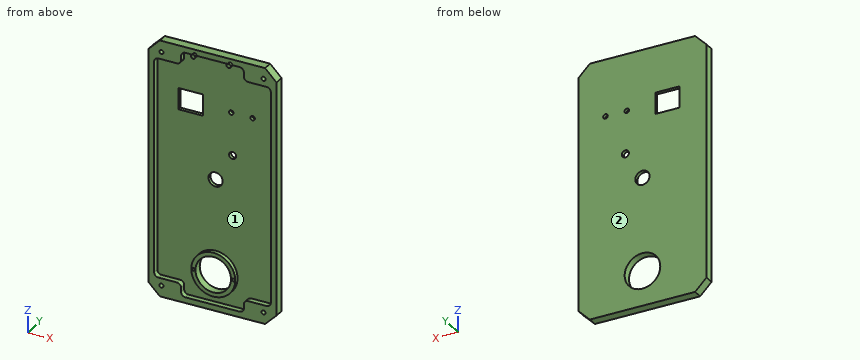
Autodesk Inventor part; units mm, degrees
ref_plane "Work Plane2" through (0, -4, 0) normal (0, -1, 0) x (1, 0, 0)
ref_plane "Work Plane1" through (0, -4, 0) normal (0, -1, 0) x (1, 0, 0)
ref_plane "YZ Plane" through (0, 0, 0) normal (1, 0, 0) x (0, 1, 0)
sketch "Sketch1" plane through (0, 0, 0) normal (0, 1, 0) x (-1, 0, 0)
  line L0 (37, -90) -> (-37, -90)
  line L1 (-45, -82) -> (-45, 82)
  line L2 (-37, 90) -> (37, 90)
  line L3 (45, 82) -> (45, -82)
  line L4 (45, -90) -> (-45, 90) construction
  line L5 (-45, -90) -> (45, 90) construction
  line L6 (-37, -90) -> (-45, -82)
  line L7 (37, -90) -> (45, -82)
  line L8 (37, 90) -> (45, 82)
  line L9 (-45, 82) -> (-37, 90)
  line L10 (0, 0) -> (0, -65.5)
  circle A0 centre (0, -65.5) radius 12.5
  line L11 (0, 0) -> (0, 0)
  circle A1 centre (0, 0) radius 5
  line L12 (0, 0) -> (17.5, 0)
  line L13 (17.5, 0) -> (17.5, 50)
  line L14 (17.5, 50) -> (0, 50)
  line L15 (0, 50) -> (0, 0)
  line L16 (26, 42.5) -> (9, 42.5)
  line L17 (9, 42.5) -> (9, 57.5)
  line L18 (9, 57.5) -> (26, 57.5)
  line L19 (26, 57.5) -> (26, 42.5)
  line L20 (26, 42.5) -> (9, 57.5) construction
  line L21 (9, 42.5) -> (26, 57.5) construction
  line L22 (9, 50) -> (-11, 50)
  circle A2 centre (-11, 50) radius 1.6
  line L23 (-11, 50) -> (-26, 50)
  circle A3 centre (-26, 50) radius 1.6
  line L24 (41, -80.3431) -> (35.3431, -86)
  line L25 (35.3431, -86) -> (-35.3431, -86)
  line L26 (-35.3431, -86) -> (-41, -80.3431)
  line L27 (-41, -80.3431) -> (-41, 80.3431)
  line L28 (-41, 80.3431) -> (-35.3431, 86)
  line L29 (-35.3431, 86) -> (35.3431, 86)
  line L30 (35.3431, 86) -> (41, 80.3431)
  line L31 (41, 80.3431) -> (41, -80.3431)
  line L32 (45, -90) -> (35.8917, -82.1873)
  circle A4 centre (35.8917, -82.1873) radius 1.45
  circle A5 centre (35.8917, -82.1873) radius 4.45
  line L33 (22.0647, -90) -> (45, -90)
  line L34 (45, -90) -> (45, -77.0647)
  line L35 (45, -77.0647) -> (22.0647, -77.0647)
  line L36 (22.0647, -77.0647) -> (22.0647, -90)
  circle A6 centre (-35.8917, -82.1873) radius 1.45
  circle A7 centre (-35.8917, -82.1873) radius 4.45
  line L37 (-45, -77.0647) -> (-22.0647, -77.0647)
  line L38 (-22.0647, -77.0647) -> (-22.0647, -90)
  circle A8 centre (35.8917, 82.1873) radius 1.45
  circle A9 centre (35.8917, 82.1873) radius 4.45
  line L39 (45, 77.0647) -> (22.0647, 77.0647)
  line L40 (22.0647, 77.0647) -> (22.0647, 90)
  circle A10 centre (-35.8917, 82.1873) radius 4.45
  circle A11 centre (-35.8917, 82.1873) radius 1.45
  line L41 (-45, 77.0647) -> (-22.0647, 77.0647)
  line L42 (-22.0647, 77.0647) -> (-22.0647, 90)
  line L43 (-22.0647, -90) -> (-45, -90)
  line L44 (-45, -90) -> (-45, -77.0647)
  line L45 (-22.0647, 90) -> (-45, 90)
  line L46 (-45, 90) -> (-45, 77.0647)
  line L47 (22.0647, 90) -> (45, 90)
  line L48 (45, 90) -> (45, 77.0647)
  line L49 (0, 0) -> (0, 20)
  line L50 (0, 0) -> (20, 0) construction
  line L51 (0, 20) -> (-12, 20)
  circle A12 centre (-12, 20) radius 2.5
  line L52 (0, 86) -> (12.5, 86)
  line L53 (0, 86) -> (-12.5, 86)
  circle A13 centre (12.5, 86) radius 1.5
  circle A14 centre (-12.5, 86) radius 1.5
  line L54 (0, -65.5) -> (14, -65.5)
  line L55 (0, -65.5) -> (14, -65.5) construction
  line L56 (0, -65.5) -> (-14, -65.5)
  line L57 (0, -65.5) -> (14, -65.5) construction
  circle A15 centre (14, -65.5) radius 0.95
  circle A16 centre (-14, -65.5) radius 0.95
  circle A17 centre (0, -65.5) radius 15.45
  point P0 (22.0647, -86)
  point P1 (-22.0647, -86)
  point P2 (-22.0647, -81.5147)
  point P3 (-26.5147, -77.0647)
  point P4 (-41, -77.0647)
  point P5 (-41, 77.0647)
  point P6 (-26.5147, 77.0647)
  point P7 (-22.0647, 81.5147)
  point P8 (-22.0647, 86)
  point P9 (22.0647, 86)
  point P10 (22.0647, 81.5147)
  point P11 (26.5147, 77.0647)
  point P12 (41, 77.0647)
  point P13 (41, -77.0647)
  point P14 (26.5147, -77.0647)
  point P15 (22.0647, -81.5147)
  point P16 (5, 0)
  point P17 (0, 5)
  point P18 (9, 50)
  point P19 (17.5, 42.5)
  dimension "d0" = 90
  dimension "d1" = 180
  dimension "d2" = 8
  dimension "d3" = 8
  dimension "d4" = 8
  dimension "d5" = 8
  dimension "d6" = 8
  dimension "d7" = 8
  dimension "d8" = 8
  dimension "d9" = 8
  dimension "d10" = 65.5
  dimension "d11" = 25
  dimension "d12" = 0
  dimension "d13" = 10
  dimension "d14" = 17.5
  dimension "d15" = 50
  dimension "d16" = 17
  dimension "d17" = 15
  dimension "d20" = 20
  dimension "d21" = 3.2
  dimension "d22" = 15
  dimension "d23" = 3.2
  dimension "d24" = 4
  dimension "d25" = 12
  dimension "d26" = 2.9
  dimension "d27" = 3
  dimension "d57" = 20
  dimension "d58" = 90
  dimension "d59" = 12
  dimension "d60" = 90
  dimension "d61" = 5
  dimension "d70" = 12.5
  dimension "d71" = 12.5
  dimension "d72" = 3
  dimension "d73" = 3
  dimension "d74" = 14
  dimension "d75" = 0
  dimension "d76" = 14
  dimension "d77" = 180
  dimension "d78" = 1.9
  dimension "d79" = 1.9
  dimension "d80" = 30.9
extrude "Extrusion1" add sketch "Sketch1" along normal blind 2.5 contours L0 L36 L25 A5 L32 L7 | L0 L38 L25 L36 | L32 A5 L24 L31 L35 L3 L7 | L0 L6 L1 L37 L27 L26 A7 L25 L38 | L36 L35 L31 L24 A5 L25 | L25 L38 L37 L27 L41 L42 L29 A14 A13 L40 L39 L31 L35 L36 | A5 L25 L24 L32 | L32 L24 A5 | L25 A7 L26 L27 L37 L38 | A4 | A5 L24 L25 | L35 L31 L39 L3 | A7 L26 L25 | L25 L26 A7 | L39 L31 L30 A9 L29 L40 L2 L8 L3 | L1 L41 L27 L37 | L39 L40 L29 A9 L30 L31 | L1 L9 L2 L42 L29 A10 L28 L27 L41 | L27 L28 A10 L29 L42 L41 | A9 L29 L30 | L30 L29 A9 | L29 A13 A14 L42 L2 L40 | A10 L29 L28 | L28 L29 A10 | A13 L29 | L29 A13 | A14 L29 | L29 A14 | A15 | A16 | A17 | A12 | A1 L15 L14 L17 L16 L13 L12 | A6 | A8 | A11
sketch "Sketch2" plane through (0, 0, 0) normal (0, -1, 0) x (1, 0, 0)
  line L0 (-26, 57.5) -> (-26, 42.5)
  line L1 (-26, 50) -> (-5, 50)
  circle A0 centre (-5, 50) radius 1.45
  circle A1 centre (-5, 50) radius 3.45
  circle A2 centre (0, -65.5) radius 12.5
  line L2 (0, -65.5) -> (-14, -65.5)
  line L3 (0, -65.5) -> (14, -65.5)
  circle A3 centre (-14, -65.5) radius 0.95
  circle A4 centre (14, -65.5) radius 0.95
  circle A5 centre (-14, -65.5) radius 1.45
  circle A6 centre (14, -65.5) radius 1.45
  line L4 (-14, -66.95) -> (-12.3751, -67.2629) construction
  line L5 (-12.3751, -67.2629) -> (-11.6091, -68.4979) construction
  spline S0 degree 2 poles (-14, -66.95) (-12.3751, -67.2629) (-11.6091, -68.4979) knots 1 1 1 2 2 2
  line L6 (-14, -64.05) -> (-12.3751, -63.7371) construction
  line L7 (-12.3751, -63.7371) -> (-11.6091, -62.5021) construction
  spline S1 degree 2 poles (-14, -64.05) (-12.3751, -63.7371) (-11.6091, -62.5021) knots 1 1 1 2 2 2
  line L8 (0, -65.5) -> (0, -61.9317)
  line L9 (14, -66.95) -> (12.3751, -67.2629) construction
  line L10 (12.3751, -67.2629) -> (11.6091, -68.4979) construction
  spline S2 degree 2 poles (14, -66.95) (12.3751, -67.2629) (11.6091, -68.4979) knots 1 1 1 2 2 2
  spline S3 degree 2 poles (14, -64.05) (12.3751, -63.7371) (11.6091, -62.5021) knots 1 1 1 2 2 2
  line L11 (14, -64.05) -> (12.3751, -63.7371) construction
  line L12 (12.3751, -63.7371) -> (11.6091, -62.5021) construction
  circle A7 centre (0, -65.5) radius 12.5
  line L13 (-22.0647, 86) -> (22.0647, 86)
  line L14 (0, 60) -> (12.5, 60)
  line L15 (12.5, 60) -> (12.5, 86)
  line L16 (12.5, 86) -> (0, 86)
  line L17 (0, 86) -> (0, 60)
  circle A8 centre (12.5, 86) radius 1.5
  circle A9 centre (-12.5, 86) radius 1.5
  circle A10 centre (0, -65.5) radius 15.45
  point P0 (0, 0)
  point P1 (-12.3047, -67.7011)
  point P2 (-12.3047, -63.2989)
  point P3 (14, -64.05)
  point P4 (12.3047, -63.2989)
  point P5 (12.3047, -67.7011)
  point P6 (-15.45, -65.5)
  point P7 (15.45, -65.5)
  dimension "d30" = 21
  dimension "d31" = 2.9
  dimension "d32" = 2
  dimension "d33" = 14
  dimension "d34" = 14
  dimension "d35" = 1.9
  dimension "d36" = 1.9
  dimension "d37" = 0.5
  dimension "d38" = 0.5
  dimension "d41" = 12.5
  dimension "d42" = 3
ref_plane "Work Plane2" through (0, -4, 0) normal (0, -1, 0) x (1, 0, 0)
sketch "Sketch4" plane through (0, -4, 0) normal (0, -1, 0) x (1, 0, 0)
  line L0 (40.0685, -6.5) -> (29.9315, -6.5)
  line L1 (29.9315, -6.5) -> (29.9315, 6.5)
  line L2 (29.9315, 6.5) -> (40.0685, 6.5)
  line L3 (40.0685, 6.5) -> (40.0685, -6.5)
  line L4 (35, 82) -> (35, -82)
  line L5 (40.0685, -6.5) -> (29.9315, 6.5) construction
  line L6 (29.9315, -6.5) -> (40.0685, 6.5) construction
  point P0 (0, 0)
  point P1 (35, 0)
  point P2 (35, -6.5)
  point P3 (35, 6.5)
  dimension "d49" = 13
ref_plane "Work Plane1" through (0, -4, 0) normal (0, -1, 0) x (1, 0, 0)
sketch "Sketch5" plane through (0, -4, 0) normal (0, -1, 0) x (1, 0, 0)
  circle A0 centre (26.5147, -81.5147) radius 1.45
  circle A1 centre (26.5147, -81.5147) radius 1.45
  circle A2 centre (-26.5147, -81.5147) radius 1.45
  circle A3 centre (-26.5147, -81.5147) radius 1.45
  circle A4 centre (26.5147, 81.5147) radius 1.45
  circle A5 centre (26.5147, 81.5147) radius 1.45
  circle A6 centre (-26.5147, 81.5147) radius 1.45
  circle A7 centre (-26.5147, 81.5147) radius 1.45
  point P0 (0, 0)
extrude "Extrusion8" add sketch "Sketch1" against normal blind 4 contours L0 L36 L25 A5 L32 L7 | L0 L38 L25 L36 | L32 A5 L24 L31 L35 L3 L7 | L0 L6 L1 L37 L27 L26 A7 L25 L38 | L36 L35 L31 L24 A5 L25 | A5 L25 L24 L32 | L32 L24 A5 | L25 A7 L26 L27 L37 L38 | A5 L24 L25 | L35 L31 L39 L3 | A7 L26 L25 | L25 L26 A7 | L39 L31 L30 A9 L29 L40 L2 L8 L3 | L1 L41 L27 L37 | L39 L40 L29 A9 L30 L31 | L1 L9 L2 L42 L29 A10 L28 L27 L41 | L27 L28 A10 L29 L42 L41 | A9 L29 L30 | L30 L29 A9 | L29 A13 A14 L42 L2 L40 | A10 L29 L28 | L28 L29 A10 | L29 A13 | A14 L29 picked at (11.5718, 86.352) picked at (-13.4282, 86.352)
extrude "Extrusion9" add sketch "Sketch2" along normal blind 3 contours L3 A6 S2 A2 | A2 S3 A6 L3 | A2 S1 A5 A10 A6 S3 | S2 A6 A10 A5 S0 A2 | A6 | A2 L2 A5 S1 | S0 A5 L2 A2 | A5
extrude "Extrusion10" cut sketch "Sketch1" along normal blind 2.5 contours L12 A1 L10 | L15 A1 L12 | L10 A1 L15
extrude "Extrusion11" cut sketch "Sketch1" against normal blind 4 contours L25 L38 L37 L27 L41 L42 L29 A14 A13 L40 L39 L31 L35 L36 | A13 L29 | L29 A14 | L12 A1 L10 | L15 A1 L12 | L10 A1 L15 | A15 | A16 | A17 picked at (11.5145, 85.8803) picked at (-13.4855, 85.8803)
extrude "Extrusion12" add sketch "Sketch1" against normal blind 3 contours A17
extrude "Extrusion13" add sketch "Sketch1" against normal blind 6 contours A13 L29 | L29 A13 | A14 L29 | L29 A14
fillet "Fillet1" radius 3 12 edges at (-41, -2, -77.0647) (-22.0647, -2, 77.0647) (22.0647, -2, -77.0647) (41, -2, -77.0647) (22.0647, -2, -86) (22.0647, -2, 77.0647) (-22.0647, -2, 86) (-41, -2, 77.0647) (41, -2, 77.0647) (22.0647, -2, 86) (-22.0647, -2, -77.0647) (-22.0647, -2, -86)
extrude "Extrusion14" cut sketch "Sketch4" against normal blind 1.5 contours L0 L1 L2 L4
extrude "Extrusion16" cut sketch "Sketch1" along normal blind 2.5 contours A12
equation "\"d3\" = d2"
equation "\"d4\" = d2"
equation "\"d5\" = d4"
equation "\"d6\" = d2"
equation "\"d7\" = d6"
equation "\"d8\" = d2"
equation "\"d9\" = d8"
properties part number "enclosed top"
Geometry: final body of the model. Coordinates: model frame, mm. Face numbers are marked on the shaded views. Coordinates: 2 decimals unless noted, no trailing zeros. Loops run counter-clockwise (first coordinate to the right, second up) from the corner with the lowest first, then second, coordinate; pieces in that order, holes last. Notation, with made-up numbers: (87.25, -10.5) - (134.25, -10.5) arc R10 ccw to (134.25, 0.5) - close; hole circle Ø7 at (21.5, 70). An arc over 180 degrees is marked (long way). One line per question, with ' | ' between items. Start each with the question number.
(1) Cut plane A-A on z = 20. Output: boundary loops of the cut face in (x, y).
(2) Draft query along X for the marked faces 1 and 2. Return one class per face: +X half, -X half, draft (parallel to the pull), parting line (faces both ways), or undercut.
(3) First-contact query: pin 1 (2.5 mm diameter, centred on x = -14, z = -65.5, fed in from -Y); pin 2 (1.5 mm diameter, centred on x = -36.5, z = -82, fed in from -Y). Flat tips, straight axial feed; report the tip coordinate or a pass-through.
(4) Cut plane D-D on z = -70.5. Output: boundary loops of the cut face in (x, y), and give its area (3 significant figures).
(5) Cut plane C-C on z = -18. Output: boundary loops of the cut face in (x, y).
(6) Ray query, L1, parallel to Z at x = 0, y = -1.3; L2, parallel to Z at x = 0, y = 1.7; L3, parallel to X at y = -1.6, z = -65.5. Return the intervals inside material, ascending. Write a range as from..to.
(7) Cut plane B-B on x = 0. Output: boundary loops of the cut face in (y, z), and give its area (3 significant figures).
Here are the results:
1) outline: (-45, -4) - (-41, -4) - (-41, 0) - (9.5, 0) - (9.5, 2.5) - (-45, 2.5) - close; (14.5, 0) - (41, 0) - (41, -4) - (45, -4) - (45, 2.5) - (14.5, 2.5) - close
2) face 1: undercut | face 2: draft
3) pin 1: y = -3 | pin 2: y = 0
4) outline: (-45, -4) - (-41, -4) - (-41, 0) - (-14.62, 0) - (-14.62, -3) - (-11.46, -3) - (-11.46, 2.5) - (-45, 2.5) - close; (11.46, -3) - (14.62, -3) - (14.62, 0) - (41, 0) - (41, -4) - (45, -4) - (45, 2.5) - (11.46, 2.5) - close | area: 219 mm²
5) outline: (-45, -4) - (-41, -4) - (-41, 0) - (41, 0) - (41, -4) - (45, -4) - (45, 2.5) - (-45, 2.5) - close
6) L1: -90..-86, -80.95..-78, -53..-50.05, 86..90 | L2: -90..-78, -53..-5, 5..90 | L3: -45..-41, -15.45..-14.95, -13.05..-12.5, 12.5..13.05, 14.95..15.45, 41..45
7) outline: (-4, -90) - (2.5, -90) - (2.5, -78) - (-3, -78) - (-3, -80.95) - (0, -80.95) - (0, -86) - (-4, -86) - close; (-4, 86) - (0, 86) - (0, 5) - (2.5, 5) - (2.5, 90) - (-4, 90) - close; (-3, -53) - (2.5, -53) - (2.5, -5) - (0, -5) - (0, -50.05) - (-3, -50.05) - close | area: 412 mm²
